Geometry: final body of the model. Coordinates: model frame, mm. A direction names the side the tool comes from. Give positions to 0.01 mm unless a question says otherwise; leave off trailing zeros. Order: outer loops, then holes, each group sorted by start corner. A loop starts at its lowest first (then second) coordinate and runs counter-clockwise, first axis right, second up. Notation, with made-up numbers: (-23, -33.5) - (-15, -33.5) arc R20 ccw to (-15, -11.5) - close; hole circle Ø6 at (51.25, -18.75). An arc over 180 degrees is marked (long way). Put each result on its own line as item: value. Start each with the question number.
1. Mould query, pull axis X, two halves, no side actions, for faces 1 (the flat face through (0, 0, 5)), 2 (the flat face through (-10, 6, 17.7)), 3 (the flat face through (11.61, 2.66, 11.26)), 4 (the flat face through (8.125, 8.732, 11.261)). Classes: pulls with the +X half, pulls with the -X half, needs draft (parallel to the pull), parting line crosses it, or undercut.
2. Section D-D on x = -6.5. Return the cut outline in (y, z), plus the area to 3 significant figures.
3. Section A-A on z = 6. Return the cut outline in (x, y), plus the area to 3 significant figures.
4. Ray query, line 1 along Y through (x, z) = (3.5, 4.25); line 2 along Z through (x, y) = (1.5, 10.75); line 3 along Y through (x, z) = (-1.5, 7.5). Return the intervals inside material, ascending. Write a range as from..to.
5. First-contact query: P1, Ø5, axis at x = 8, y = -4.5, coming from the +Z side; P2, Ø0.5, axis at y = -11, z = 10, coming from the -X side; P3, Ø0.8, axis at x = 0, z = 10.5, coming from the -Y side. Flat tips, straight axial feed; report the tip coordinate or a pass-through.
6. Set-up query: faces 5 (the flat face through (3.5, -11.4, 11.3)), 6 (the cylindrical face through (-9.936, 5.679, 11.261)), 7 (the cylindrical face through (0.433, -12.392, 2.465)). Return all of +Z, -Z, +X, -X, +Y, -Y with unobstructed straight access to the full face (end or side cutting, diameter ignored); none if empty.
7. Section C-C on y = 12. Return the cut outline in (x, z).
from build123d import *

# Parameters (mm, degrees)
SKETCH2_W              = 26.816018719
SKETCH2_H              = 28.301670726
SQUARE_EXTRUDE_DEPTH   = 5
ACTUAL_SHAPE_CUT_DEPTH = 5
SKETCH3_W              = 14.9
SKETCH3_H              = 3.687507881
STOPPERS_EXTRUDE_DEPTH = 12.7
CURVE_CUT_DEPTH        = 12.7


with BuildPart() as part:
    # Sketch2 → Square extrude (new body)
    with BuildSketch(Plane.XY):
        with Locations((0.074282601, 0.767135851)):
            Rectangle(SKETCH2_W, SKETCH2_H)
    extrude(amount=SQUARE_EXTRUDE_DEPTH)

    # Sketch1 → Actual shape cut (cut)
    with BuildSketch(Plane.XY):
        with BuildLine():
            Line((-17.45, 14.04483891), (-17.45, 23.6))
            Line((-17.45, 23.6), (17.45, 23.6))
            Line((17.45, 23.6), (17.45, 14.04483891))
            ThreePointArc((17.45, 14.04483891), (0, -22.4), (-17.45, 14.04483891))
        make_face()
        with BuildLine():
            Line((-7.45, 9.912492119), (-7.45, 13.6))
            Line((-7.45, 13.6), (7.45, 13.6))
            Line((7.45, 13.6), (7.45, 9.912492119))
            ThreePointArc((7.45, 9.912492119), (0, -12.4), (-7.45, 9.912492119))
        make_face(mode=Mode.SUBTRACT)
    extrude(amount=ACTUAL_SHAPE_CUT_DEPTH, mode=Mode.SUBTRACT)

    # Sketch3 → Stoppers extrude (add)
    with BuildSketch(Plane.XY.offset(5)):
        with Locations((0, 11.75624606)):
            Rectangle(SKETCH3_W, SKETCH3_H)
        with BuildLine():
            Line((3.5, -11.895797577), (3.5, -10.895797577))
            ThreePointArc((3.5, -10.895797577), (0, -11.444142818), (-3.5, -10.895797577))
            Line((-3.5, -10.895797577), (-3.5, -11.895797577))
            Line((-3.5, -11.895797577), (-2.187402084, -12.20554268))
            Line((-2.187402084, -12.20554268), (-0.759747946, -12.376703239))
            Line((-0.759747946, -12.376703239), (0.759747946, -12.376703239))
            Line((0.759747946, -12.376703239), (2.226876894, -12.198402326))
            Line((2.226876894, -12.198402326), (3.5, -11.895797577))
        make_face()
        with BuildLine():
            Line((-12.0520629, 2.916809875), (-11.186037496, 2.416809875))
            ThreePointArc((-11.186037496, 2.416809875), (-9.910918405, 5.722071409), (-7.686037496, 8.478987702))
            Line((-7.686037496, 8.478987702), (-8.5520629, 8.978987702))
            Line((-8.5520629, 8.978987702), (-9.476608986, 7.997117113))
            Line((-9.476608986, 7.997117113), (-10.338665447, 6.846312641))
            Line((-10.338665447, 6.846312641), (-11.098413393, 5.530390597))
            Line((-11.098413393, 5.530390597), (-11.677564746, 4.170669202))
            Line((-11.677564746, 4.170669202), (-12.0520629, 2.916809875))
        make_face()
        with BuildLine():
            Line((8.5520629, 8.978987702), (7.686037496, 8.478987702))
            ThreePointArc((7.686037496, 8.478987702), (9.910918405, 5.722071409), (11.186037496, 2.416809875))
            Line((11.186037496, 2.416809875), (12.0520629, 2.916809875))
            Line((12.0520629, 2.916809875), (11.66401107, 4.208425567))
            Line((11.66401107, 4.208425567), (11.098413393, 5.530390597))
            Line((11.098413393, 5.530390597), (10.338665447, 6.846312641))
            Line((10.338665447, 6.846312641), (9.450687853, 8.027733124))
            Line((9.450687853, 8.027733124), (8.5520629, 8.978987702))
        make_face()
    extrude(amount=STOPPERS_EXTRUDE_DEPTH)

    # Sketch4 → Curve cut (cut)
    with BuildSketch(Plane.XY.offset(17.7)):
        with BuildLine():
            Line((-7.45, 9.912492119), (7.45, 9.912492119))
            ThreePointArc((7.45, 9.912492119), (0, 12.4), (-7.45, 9.912492119))
        make_face()
    extrude(amount=-CURVE_CUT_DEPTH, mode=Mode.SUBTRACT)


solid = part.part
Resolved:
1. face 1: undercut
1. face 2: needs draft
1. face 3: pulls with the +X half
1. face 4: undercut
2. outline: (-10.56, 0) - (13.6, 0) - (13.6, 17.7) - (10.56, 17.7) - (10.56, 5) - (-10.56, 5) - close
2. area: 159 mm^2
3. outline: (-12.05, 2.92) - (-11.19, 2.42) arc R11.44 cw to (-7.69, 8.48) - (-8.55, 8.98) - (-9.48, 8) - (-10.34, 6.85) - (-11.1, 5.53) - (-11.68, 4.17) - close; (-7.45, 9.91) arc R12.4 cw to (7.45, 9.91) - (7.45, 13.6) - (-7.45, 13.6) - close; (-3.5, -11.9) - (-2.19, -12.21) - (-0.76, -12.38) - (0.76, -12.38) - (2.23, -12.2) - (3.5, -11.9) - (3.5, -10.9) arc R11.44 cw to (-3.5, -10.9) - close; (7.69, 8.48) arc R11.44 cw to (11.19, 2.42) - (12.05, 2.92) - (11.66, 4.21) - (11.1, 5.53) - (10.34, 6.85) - (9.45, 8.03) - (8.55, 8.98) - close
3. area: 49.8 mm^2
4. line 1: -11.9..13.6
4. line 2: 0..5
4. line 3: -12.29..-11.35, 12.31..13.6
5. P1: z = 5
5. P2: x = -3.5
5. P3: y = -12.38
6. face 5: +Z, +X, -Y
6. face 6: +Z, -Y
6. face 7: +Z, -Z
7. outline: (-7.45, 0) - (7.45, 0) - (7.45, 17.7) - (3.12, 17.7) - (3.12, 5) - (-3.12, 5) - (-3.12, 17.7) - (-7.45, 17.7) - close
